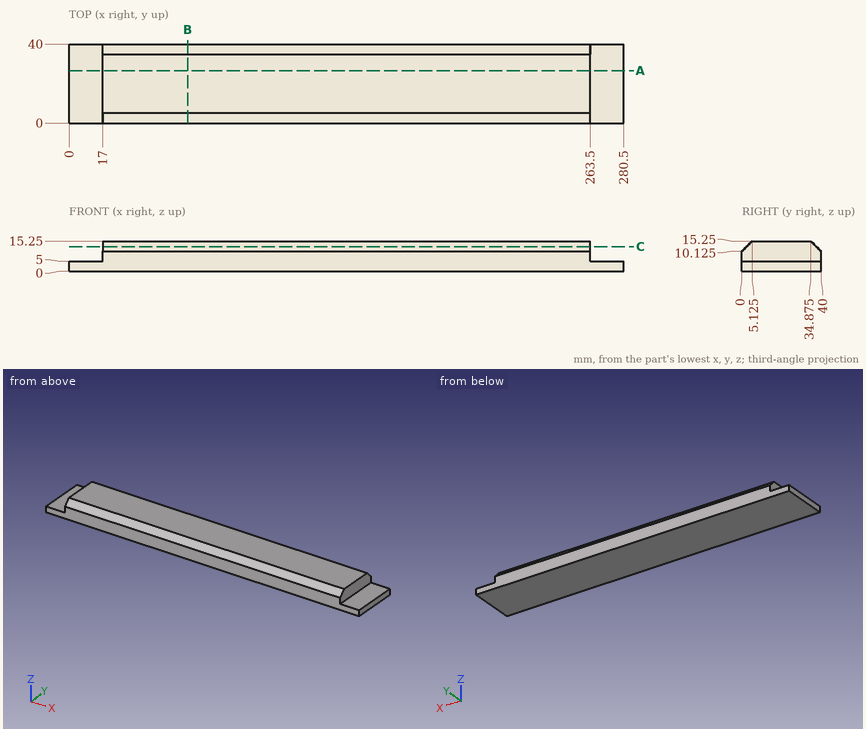
Design review of the part shown in the three views and the two pictorial views. Dimensions are in mm from the part's minimum x, y and z. Round coordinates to 2 decimals unless told otherwise and drop trailing zeros. Write each loop counter-clockwise with the first axis right and the second up, starting at its lowest first coordinate (ties: lowest second). Pieces come first, ordered by that corner, then holes. Notation, with made-up numbers: (78.25, 1.25) - (104.25, 1.25) arc R16 cw to (104.25, 28.25) - close; hole circle Ø5 at (-38.5, 78). An arc over 180 degrees is marked (long way). Answer as CSV lines item,"result". Start each with the question number.
(1) For line 1 (X direction, y = 9, z = 12); line 2 (Z direction, x = 102.5, y = 36) (3 decimals); line 3 (Z direction, x = 47, y = 5) (3 decimals), list the stretches that pass through material, from the lowest coordinate up.
(2) Add section C-C, the plane z = 12.5. State the section outline as (x, y) points (3 decimals).
(3) Add section B-B, the plane x = 60. State the section outline as (y, z) points (3 decimals).
(4) For pin 1 (5 mm diameter, centred on y = 11, z = 8, fed in from -X); pin 2 (5 mm diameter, centred on x = 7, y = 15, fed in from +Z); pin 3 (6 mm diameter, centred on x = 35.5, y = 23, fed in from -Z); pin 4 (2 mm diameter, centred on x = 244, z = 11.5, fed in from -Y) (3 decimals), all flat-tipped, find the tip position at first contact; note any pin that passes through.
(5) Add section A-A, the plane y = 26.5. State the section outline as (x, z) points.
From the geometry:
1,line 1,"x = 17 to 263.5"
1,line 2,"z = 0 to 14.125"
1,line 3,"z = 0 to 15.125"
2,outline,"(17, 2.375) - (263.5, 2.375) - (263.5, 37.625) - (17, 37.625) - close"
3,outline,"(0, 0) - (40, 0) - (40, 10.125) - (34.875, 15.25) - (5.125, 15.25) - (0, 10.125) - close"
4,pin 1,"stops at x = 17"
4,pin 2,"stops at z = 5"
4,pin 3,"stops at z = 0"
4,pin 4,"stops at y = 0.375"
5,outline,"(0, 0) - (280.5, 0) - (280.5, 5) - (263.5, 5) - (263.5, 15.25) - (17, 15.25) - (17, 5) - (0, 5) - close"
